CAD build for the part. Positions are in the model's coordinates, mm. A direction names the side the tool comes from. Round coordinates to 2 decimals unless told otherwise and drop trailing zeros. Order: outer loops, then holes, each group sorted by start corner. A loop starts at its lowest first (then second) coordinate and runs counter-clockwise, first axis right, second up. Notation, with made-up numbers: M 4,-13.75 L 28,-13.75 A17 cw 28,0.25 Z; hole C -19,34 d9. An arc over 180 degrees is marked long. Answer as CSV lines item,"result". Start each with the question number.
```python
from build123d import *

# Parameters (mm, degrees)
SKETCH1_R                = 4
IMPELLER_SECTION_DEPTH   = 10.2921875
SKETCH2_R                = 2
IMPELLER_BOLT_BORE_DEPTH = 6.2921875
SEAL_START               = 26.0921875
SKETCH3_R                = 4
SEAL_SECTION_DEPTH       = 26.0921875
DOWEL_HOLE_DEPTH         = 10
DOWEL_HOLE_DEPTH_BACK    = 10
SKETCH5_R                = 1
SKETCH6_R                = 6
BEARING_STOP_DEPTH       = 2
SKETCH8_R                = 5
BEARING_SECTION_DEPTH    = 10
BOSS_EXTRUDE4_START      = 18.5
SKETCH9_R                = 4
BOSS_EXTRUDE4_DEPTH      = 18.5


with BuildPart() as part:
    # Sketch1 → impeller section (new body)
    with BuildSketch(Plane(origin=(0, 0, 0), x_dir=(1, 0, 0), z_dir=(0, 1, 0))):
        with Locations(Location((0, 0, 0), (0, 0, 270))):
            Circle(SKETCH1_R)
    extrude(amount=IMPELLER_SECTION_DEPTH)

    # Sketch2 → impeller bolt bore (cut)
    with BuildSketch(Plane(origin=(0, 10.2921875, 0), x_dir=(1, 0, 0), z_dir=(0, 1, 0))):
        with Locations(Location((0, 0, 0), (0, 0, 270))):
            Circle(SKETCH2_R)
    extrude(amount=-IMPELLER_BOLT_BORE_DEPTH, mode=Mode.SUBTRACT)

    # Sketch3 → seal section (add)
    with BuildSketch(Plane(origin=(0, 0, 0), x_dir=(-1, 0, 0), z_dir=(0, -1, 0)).offset(SEAL_START)):
        with Locations(Location((0, 0, 0), (0, 0, 90))):
            Circle(SKETCH3_R)
    extrude(amount=-SEAL_SECTION_DEPTH)

    # Sketch5 → dowel hole (cut, two sides: drawn at the far end of the back side and taken through both)
    with BuildSketch(Plane(origin=(0, 0, 0), x_dir=(0, 0, -1), z_dir=(1, 0, 0)).offset(-DOWEL_HOLE_DEPTH_BACK)):
        with Locations(Location((0, 1, 0), (0, 0, 180))):
            Circle(SKETCH5_R)
    extrude(amount=DOWEL_HOLE_DEPTH + DOWEL_HOLE_DEPTH_BACK, mode=Mode.SUBTRACT)

    # Sketch6 → bearing stop (add)
    with BuildSketch(Plane.XZ.offset(26.0921875)):
        with Locations(Location((0, 0, 0), (0, 0, 270))):
            Circle(SKETCH6_R)
    extrude(amount=BEARING_STOP_DEPTH)

    # Sketch8 → bearing section (add)
    with BuildSketch(Plane.XZ.offset(28.0921875)):
        with Locations(Location((0, 0, 0), (0, 0, 270))):
            Circle(SKETCH8_R)
    extrude(amount=BEARING_SECTION_DEPTH)

    # Sketch9 → Boss-Extrude4 (add)
    with BuildSketch(Plane(origin=(0, -38.0921875, 0), x_dir=(-1, 0, 0), z_dir=(0, -1, 0)).offset(BOSS_EXTRUDE4_START)):
        with Locations(Location((0, 0, 0), (0, 0, 90))):
            Circle(SKETCH9_R)
    extrude(amount=-BOSS_EXTRUDE4_DEPTH)


solid = part.part
```
Q1. Band-saw the part on D-D, the plane y = -40. Write the cut outline in (x, z).
Q2. Drop flat-ended pins along their axis: P1, Ø4, axis at x = 1.5, y = -42.5, coming from the -Z side; P2, Ø1.5, axis at x = -0.5, y = -42, coming from the +Z side; P3, Ø1.5, axis at x = 2, y = -30, coming from the -Z side; P4, Ø1.2, axis at y = 1, z = 0, coming from the -X side. Give the stop position or say it passes through.
Q3. Band-saw the part on B-B, the plane x = 0. Write the cut outline in (y, z).
Q4. Mould opens along Z. For faces 4 (the flat face through (0, 4, 0)), 5 (the cylindrical face through (-4.88, -33.02, 1.08)), 6 (the flat face through (-1, 10.292, -2)) say: +Z half, -Z half, draft (parallel to the pull), parting line (faces both ways), or undercut.
Q5. Band-saw the part on C-C, the plane y = 1. Write the cut outline in (x, z).
Q6. Band-saw the part on A-A, the plane z = 0. Write the cut outline in (x, y).
Q7. Probe line 1 along Y through (x, z) = (-2.25, 0); line 2 along Y through (x, z) = (1, 0); line 3 along X through (y, z) = (6.25, 0). List the from-to ranges inside material, lowest first. Write a range as from..to.
Q8. Tool access for faces 1 (the flat face through (-3.92, -26.092, 1.42)), 2 (the flat face through (0, -56.592, 0)), 3 (the flat face through (4, -28.092, 4)): list every direction of +Z, -Z, +X, -X, +Y, -Y with a clear straight run to the whole face (end or side of a thin tool).
Answer:
1,outline,"C 0,0 d8"
2,P1,"stops at z = -4"
2,P2,"stops at z = 4"
2,P3,"stops at z = -4.84"
2,P4,"passes through"
3,outline,"M -56.59,-4 L -38.09,-4 L -38.09,-5 L -28.09,-5 L -28.09,-6 L -26.09,-6 L -26.09,-4 L 10.29,-4 L 10.29,-2 L 4,-2 L 4,2 L 10.29,2 L 10.29,4 L -26.09,4 L -26.09,6 L -28.09,6 L -28.09,5 L -38.09,5 L -38.09,4 L -56.59,4 Z; hole C 1,0 d2"
4,face 4,"undercut"
4,face 5,"parting line"
4,face 6,"draft"
5,outline,"M -3.87,-1 A4 ccw 3.87,-1 Z; M -3.87,1 L 3.87,1 A4 ccw Z"
6,outline,"M -6,-28.09 L -5,-28.09 L -5,-38.09 L -4,-38.09 L -4,-56.59 L 4,-56.59 L 4,-38.09 L 5,-38.09 L 5,-28.09 L 6,-28.09 L 6,-26.09 L 4,-26.09 L 4,0 L -4,0 L -4,-26.09 L -6,-26.09 Z; M -4,2 L 4,2 L 4,10.29 L 2,10.29 L 2,4 L -2,4 L -2,10.29 L -4,10.29 Z"
7,line 1,"y = -56.59..0, 2..10.29"
7,line 2,"y = -56.59..0, 2..4"
7,line 3,"x = -4..-2, 2..4"
8,face 1,"+Y"
8,face 2,"+Z, -Z, +X, -X, -Y"
8,face 3,"-Y"
